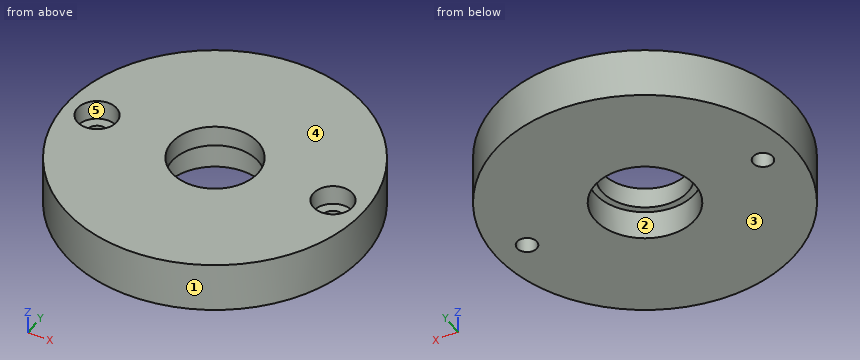
from build123d import *

# Parameters (mm, degrees)
ESQUISSE1_R             = 38.1
ESQUISSE1_R_2           = 11
BOSS_EXTRU_1_DEPTH      = 12.7
ESQUISSE2_R             = 12.7
ENL_V_MAT_EXTRU_1_DEPTH = 7.4
ESQUISSE3_R             = 2.5
ENL_V_MAT_EXTRU_2_DEPTH = 13.7
ESQUISSE4_R             = 5
ENL_V_MAT_EXTRU_3_DEPTH = 5


with BuildPart() as part:
    # Esquisse1 → Boss.-Extru.1 (new body)
    with BuildSketch(Plane.XY):
        with Locations((23.012291104, 8.435887891)):
            Circle(ESQUISSE1_R)
        with Locations((23.012291104, 8.435887891)):
            Circle(ESQUISSE1_R_2, mode=Mode.SUBTRACT)
    extrude(amount=BOSS_EXTRU_1_DEPTH)

    # Esquisse2 → Enlèv. mat.-Extru.1 (cut)
    with BuildSketch(Plane(origin=(0, 0, 0), x_dir=(-1, 0, 0), z_dir=(0, 0, -1))):
        with Locations((-23.012291104, 8.435887891)):
            Circle(ESQUISSE2_R)
    extrude(amount=-ENL_V_MAT_EXTRU_1_DEPTH, mode=Mode.SUBTRACT)

    # Esquisse3 → Enlèv. mat.-Extru.2 (cut, through all)
    with BuildSketch(Plane.XY.offset(12.7)):
        with Locations((53.174791104, 8.435887891)):
            Circle(ESQUISSE3_R)
        with Locations((-7.150208896, 8.435887891)):
            Circle(ESQUISSE3_R)
    extrude(amount=-ENL_V_MAT_EXTRU_2_DEPTH, mode=Mode.SUBTRACT)

    # Esquisse4 → Enlèv. mat.-Extru.3 (cut)
    with BuildSketch(Plane.XY.offset(12.7)):
        with Locations((-7.150208896, 8.435887891)):
            Circle(ESQUISSE4_R)
        with Locations((53.174791104, 8.435887891)):
            Circle(ESQUISSE4_R)
    extrude(amount=-ENL_V_MAT_EXTRU_3_DEPTH, mode=Mode.SUBTRACT)


solid = part.part
Input: part model. Units: mm. Frame: model coordinates. Face numbers are marked on the shaded views. A direction names the side the tool comes from. Round coordinates to 2 decimals unless told otherwise and drop trailing zeros. Order: outer loops, then holes, each group sorted by start corner. A loop starts at its lowest first (then second) coordinate and runs counter-clockwise, first axis right, second up. Notation, with made-up numbers: (32.25, 84.5) - (62.25, 84.5) arc R25 cw to (62.25, 118.5) - close; hole circle Ø10 at (1.5, 29). An arc over 180 degrees is marked (long way). Use a Markdown table: item, result.
1. Section A-A on x = 13. Return the cut outline in (y, z).
Evaluation:
| item | result |
|---|---|
| outline | (-28.33, 0) - (0.62, 0) - (0.62, 7.4) - (3.88, 7.4) - (3.88, 12.7) - (-28.33, 12.7) - close; (12.99, 7.4) - (16.25, 7.4) - (16.25, 0) - (45.2, 0) - (45.2, 12.7) - (12.99, 12.7) - close |
2. Access query for the marked faces 4 and 5. Directions: +Z, -Z, +X, -X, +Y, -Y. A direction counts if a zero-diameter tool reaches every point of the face in a straight line with its end or side. Return the directions, or none.
Evaluation:
| item | result |
|---|---|
| face 4 | +Z, +X, -X, +Y, -Y |
| face 5 | +Z |
3. Section C-C on z = 3.5. Return the cut outline in (x, y).
Evaluation:
| item | result |
|---|---|
| outline | circle Ø76.2 at (23.01, 8.44); hole circle Ø5 at (-7.15, 8.44); hole circle Ø25.4 at (23.01, 8.44); hole circle Ø5 at (53.17, 8.44) |
4. First-contact query: pin 1 (6 mm diameter, centred on x = 38, z = 8.5, fed in from -Y); pin 2 (4 mm diameter, centred on x = 42.5, z = 6, fed in from +Y). Flat tips, straight axial feed; report the tip coordinate or a pass-through.
Evaluation:
| item | result |
|---|---|
| pin 1 | y = -27.73 |
| pin 2 | y = 42.29 |
5. Mould query, pull axis X, two halves, no side actions, for the marked faces 1, 2 and 3. Classes: +X half, -X half, draft (parallel to the pull), parting line (faces both ways), or undercut.
Evaluation:
| item | result |
|---|---|
| face 1 | parting line |
| face 2 | undercut |
| face 3 | draft |
6. Material intervals for probe 1 along Y at (x, z) = (52, 1.5); probe 2 along Y at (x, z) = (16, 10.75); probe 3 along X at (y, z) = (5, 1.75), sorted ascending.
Evaluation:
| item | result |
|---|---|
| probe 1 | -16.29 to 6.23, 10.64 to 33.16 |
| probe 2 | -29.01 to -0.04, 16.91 to 45.89 |
| probe 3 | -14.93 to 10.79, 35.24 to 60.96 |
7. Section B-B on y = 0.5. Return the cut outline in (x, z).
Evaluation:
| item | result |
|---|---|
| outline | (-14.25, 0) - (13.1, 0) - (13.1, 7.4) - (15.4, 7.4) - (15.4, 12.7) - (-14.25, 12.7) - close; (30.63, 7.4) - (32.93, 7.4) - (32.93, 0) - (60.28, 0) - (60.28, 12.7) - (30.63, 12.7) - close |
8. Section D-D on y = 27.5. Return the cut outline in (x, z), then the cut area to 3 significant figures.
Evaluation:
| item | result |
|---|---|
| outline | (-9.98, 0) - (56, 0) - (56, 12.7) - (-9.98, 12.7) - close |
| area | 838 mm^2 |
